Here's how the part is built. I have some questions about the finished solid (model axes, mm). A direction names the side the tool comes from. Coordinates: 2 decimals unless noted, no trailing zeros. Loops run counter-clockwise (first coordinate to the right, second up) from the corner with the lowest first, then second, coordinate; pieces in that order, holes last. Notation, with made-up numbers: (-11, 23) -> (21, 23) arc R14 cw to (21, 33) -> close; hole circle Ø7 at (-7.5, 19.5). An arc over 180 degrees is marked (long way). Answer as a JSON object with one key per item and string values. Group by question number.
1) I want a section at B-B (x = 0). Write out the boundary of the cut face in (y, z), then the cut area to 3 significant figures.
2) I want a section at D-D (z = 6.5). Write out the boundary of the cut face in (x, y), then the cut area to 3 significant figures.
3) I'm going to push a flat-ended pin straight in: pin 1 (2.5 mm diameter, centred on x = 0.5, y = 0.5, fed in from -Z). Where does the tip first touch, or does it pass through?
4) I want a section at A-A (z = 3). Write out the boundary of the cut face in (x, y), then the cut area to 3 significant figures.
5) Which directions (+Z, -Z, +X, -X, +Y, -Y) give clear straight access to the entire face, cutting with the end or side of a thin tool? Please do faces 4 (the flat face through (0, -2.8, 3)), 5 (the flat face through (0, 0, 5)).
6) If we mould it in two halves opening along X, with no side actions, what happens to faces 1 (the flat face through (1.4, 1.3, 0)), 2 (the flat face through (-2.436, -1.38, 3.451)), 3 (the cylindrical face through (-1.27, -0.97, 2.46))? For each: +X half, -X half, draft (parallel to the pull), parting line (faces both ways), or undercut.
7) I need wall thicknesses on probe 1 along Y at (x, z) = (0, 2.8); probe 2 along Y at (x, z) = (1, 2.25); probe 3 along X at (y, z) = (1.3, 3.25). Which ranges of each line are inside material? Lowest first, please. Write a range as [from, to].
8) I want a section at C-C (y = -0.25). Write out the boundary of the cut face in (x, z), then the cut area to 3 significant figures.
```python
from build123d import *

# Parameters (mm, degrees)
F2_R     = 1.6
F3_DEPTH = 5
F4_R     = 1.6
F5_DEPTH = 2


with BuildPart() as f3:
    # F2 (on Top) → F3 (new body)
    with BuildSketch(Plane.XY):
        Polygon((-1.6165807537, -2.8), (1.6165807537, -2.8), (3.2331615075, 0), (1.6165807537, 2.8), (-1.6165807537, 2.8), (-3.2331615075, 0), align=None)
        Circle(F2_R, mode=Mode.SUBTRACT)
    extrude(amount=F3_DEPTH)

    # F4 (on face) → F5 (join)
    with BuildSketch(Plane.XY.offset(5)):
        Polygon((-1.6165807537, -2.8), (1.6165807537, -2.8), (3.2331615075, 0), (1.6165807537, 2.8), (-1.6165807537, 2.8), (-3.2331615075, 0), align=None)
        Circle(F4_R, mode=Mode.SUBTRACT)
        Circle(F4_R)
    extrude(amount=F5_DEPTH)


solid = f3.part
```
Determined:
{
 "1": {"outline": "(-2.8, 0) -> (-1.6, 0) -> (-1.6, 5) -> (1.6, 5) -> (1.6, 0) -> (2.8, 0) -> (2.8, 7) -> (-2.8, 7) -> close", "area": "23.2 mm^2"},
 "2": {"outline": "(-3.23, 0) -> (-1.62, -2.8) -> (1.62, -2.8) -> (3.23, 0) -> (1.62, 2.8) -> (-1.62, 2.8) -> close", "area": "27.2 mm^2"},
 "3": {"pin 1": "z = 0"},
 "4": {"outline": "(-3.23, 0) -> (-1.62, -2.8) -> (1.62, -2.8) -> (3.23, 0) -> (1.62, 2.8) -> (-1.62, 2.8) -> close; hole circle Ø3.2 at (0, 0)", "area": "19.1 mm^2"},
 "5": {"face 4": "+Z, -Z, +X, -X, -Y", "face 5": "-Z"},
 "6": {"face 1": "draft", "face 2": "-X half", "face 3": "undercut"},
 "7": {"probe 1": "[-2.8, -1.6], [1.6, 2.8]", "probe 2": "[-2.8, -1.25], [1.25, 2.8]", "probe 3": "[-2.48, -0.93], [0.93, 2.48]"},
 "8": {"outline": "(-3.09, 0) -> (-1.58, 0) -> (-1.58, 5) -> (1.58, 5) -> (1.58, 0) -> (3.09, 0) -> (3.09, 7) -> (-3.09, 7) -> close", "area": "27.4 mm^2"}
}
